Geometry: final body of the model. Coordinates: model frame, mm. Coordinates: 2 decimals unless noted, no trailing zeros. Order: outer loops, then holes, each group sorted by start corner. A loop starts at its lowest first (then second) coordinate and runs counter-clockwise, first axis right, second up. Notation, with made-up numbers: M 2,6 L 7,6 A25 ccw 7,20 Z; hole C 38.25,48.5 d11. An arc over 180 degrees is marked long. One line per question, with ' | ' between items.
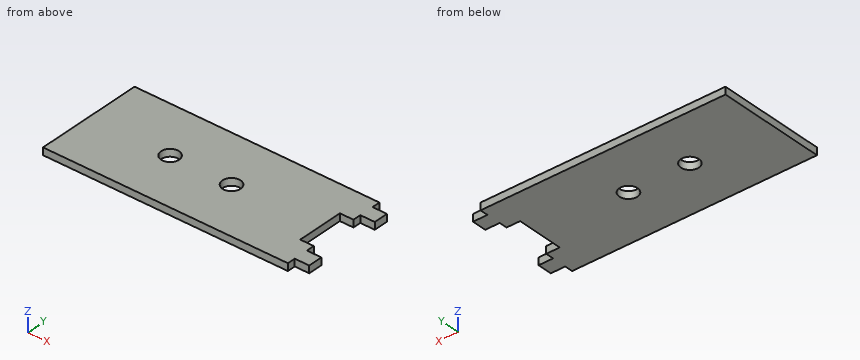
from build123d import *

# Parameters (mm, degrees)
SKETCH1_R           = 5
BOSS_EXTRUDE1_DEPTH = 4


with BuildPart() as part:
    # Sketch1 → Boss-Extrude1 (new body)
    with BuildSketch(Plane.XY):
        Polygon((49, 30), (56.5, 30), (56.5, 25.5), (64.5, 25.5), (64.5, 17.5), (56.5, 17.5), (56.5, 13), (49, 13), (49, -13), (56.5, -13), (56.5, -17.5), (64.5, -17.5), (64.5, -25.5), (56.5, -25.5), (56.5, -30), (49, -30), (-79, -30), (-79, 30), align=None)
        Circle(SKETCH1_R, mode=Mode.SUBTRACT)
        with Locations((-34, 0)):
            Circle(SKETCH1_R, mode=Mode.SUBTRACT)
    extrude(amount=BOSS_EXTRUDE1_DEPTH)


solid = part.part
1. Section A-A, the plane x = -34. Output: boundary loops of the cut face in (y, z).
Response values:
outline: M -30,0 L -5,0 L -5,4 L -30,4 Z; M 5,0 L 30,0 L 30,4 L 5,4 Z
2. Material intervals for line 1 (Y direction, x = -34.5, z = 0.7); line 2 (X direction, y = -3, z = 0.6); line 3 (X direction, y = 14, z = 0.3), sorted ascending. Write a range as [from, to].
Response values:
line 1: y = [-30, -4.97], [4.97, 30] | line 2: x = [-79, -38], [-30, -4], [4, 49] | line 3: x = [-79, 56.5]
3. Pin query (flat end, axial travel): P1, Ø1.2, axis at y = -15, z = 3, coming from the +X side; P2, Ø13, axis at x = -34, y = 0, coming from the -Z side; P3, Ø1.2, axis at x = 61, z = 2, coming from the +Y side. Return the tip coordinate at first contact, or that it passes through.
Response values:
P1: stops at x = 56.5 | P2: stops at z = 0 | P3: stops at y = 25.5
4. Section B-B, the plane z = 1.25. Output: boundary loops of the cut face in (x, y), and give its area (3 significant figures).
Response values:
outline: M -79,-30 L 56.5,-30 L 56.5,-25.5 L 64.5,-25.5 L 64.5,-17.5 L 56.5,-17.5 L 56.5,-13 L 49,-13 L 49,13 L 56.5,13 L 56.5,17.5 L 64.5,17.5 L 64.5,25.5 L 56.5,25.5 L 56.5,30 L -79,30 Z; hole C -34,0 d10; hole C 0,0 d10 | area: 7,910 mm^2
5. Section C-C, the plane y = -7.5. Output: boundary loops of the cut face in (x, z).
Response values:
outline: M -79,0 L 49,0 L 49,4 L -79,4 Z
